The model under review builds one solid part; all positions refer to its coordinate system, in mm. A direction names the side the tool comes from. Round coordinates to 2 decimals unless told otherwise and drop trailing zeros. Write each loop counter-clockwise with the first axis right and the second up, starting at its lowest first coordinate (ties: lowest second). Pieces come first, ordered by that corner, then holes. Notation, with made-up numbers: (79, -21.75) -> (99, -21.75) arc R17 ccw to (99, 5.25) -> close; hole circle Ø10 at (81, -16). An arc over 180 degrees is marked (long way). Use CSV: the item, a comma, the result in double quotes. Start each with the question number.
1) Machinability: for faces 1 (the face through (29, 9, -4.8)), 2 (the face through (15, 2, -10)), 3 (the face through (-27.8, 2.74, 7.27)), which of the approach directions +Z, -Z, +X, -X, +Y, -Y give a long, thin tool a straight path to every point of the face, cutting with its end or side? Answer none if there is none.
2) Mouldability with a two-part tool opening along Z and no side actions: class faces 4 (the face through (-14.75, 0.56, -9.58)), 5 (the face through (-29.88, 14.56, -7.84)) as released by +Z, released by -Z, zero draft, split by the parting line, or undercut.
3) Take a section at C-C, the plane z = 17. Give the boundary of the cut face in (x, y).
4) For pin 1 Ø6 at (y, z) = (22, -5) entering from +X; pin 2 Ø5 at (x, z) = (-26, -3.5) entering from +Y; pin 3 Ø2.5 at (x, z) = (0, -8) entering from +Y; pin 4 Ø8 at (x, z) = (6, 9.5) entering from +Y, all flat-tipped, find the tip position at first contact; note any pin that passes through.
5) Wall thickness on probe 1 along Z at (x, y) = (0, 14); probe 2 along Z at (x, y) = (-22, 10); probe 3 along X at (y, z) = (9.5, -10.5): over which ranges is each line inside the solid? List them lowest first. Write a range as [from, to].
6) Take a section at D-D, the plane z = 12. Give the boundary of the cut face in (x, y).
7) Take a section at B-B, the plane y = 15. Give the boundary of the cut face in (x, z).
8) Take a section at A-A, the plane x = 0. Give the boundary of the cut face in (y, z).
from build123d import *

# Parameters (mm, degrees)
EXTRUDE_1_DEPTH     = 25
EXTRUDE_2_DEPTH     = 36
SKETCH_3_W          = 15
SKETCH_3_H          = 6
EXTRUDE_3_DEPTH     = 12
SKETCH_4_R          = 0.95
CUT_EXTRUDE_1_DEPTH = 21
SKETCH_5_R          = 4
SKETCH_5_R_2        = 1.45
EXTRUDE_4_DEPTH     = 23
SKETCH_6_R          = 1.75
CUT_EXTRUDE_2_DEPTH = 20
SKETCH_7_R          = 2.5
CUT_EXTRUDE_3_DEPTH = 2
CUT_EXTRUDE_4_DEPTH = 53.393911874
FILLET_4_R          = 1


with BuildPart() as part:
    # 草图1 → 凸台-拉伸1 (new, symmetric)
    with BuildSketch(Plane.XY):
        Polygon((0, 0), (9.650045346, 0), (39.194277936, -5.20944533), (39.888870647, -1.270214318), (10, 4), (0, 4), align=None)
    extrude_1 = extrude(amount=EXTRUDE_1_DEPTH, both=True)

    # 草图2 → 凸台-拉伸2 (add)
    with BuildSketch(Plane.XY.offset(25)):
        Polygon((20.192715587, 2.202749235), (20.513964715, 4.024643578), (35.286081011, 1.419920913), (34.964831882, -0.40197343), align=None)
    extrude_2 = extrude(amount=-EXTRUDE_2_DEPTH)

    # 草图3 → 凸台-拉伸3 (add)
    with BuildSketch(Plane(origin=(1.306826311, 7.411380301, 0), x_dir=(0.9848077530122079, -0.1736481776669312, 0), z_dir=(0.1736481776669312, 0.9848077530122079, 0))):
        with Locations((27.003439474, -22)):
            Rectangle(SKETCH_3_W, SKETCH_3_H)
        with Locations((27.003439474, 7.8)):
            Rectangle(SKETCH_3_W, SKETCH_3_H)
    extrude_3 = extrude(amount=EXTRUDE_3_DEPTH)

    # 草图4 → 切除-拉伸1 (cut)
    with BuildSketch(Plane(origin=(33.979254699, -5.991459388, 0), x_dir=(0, 0, -1), z_dir=(0.9848077530122081, -0.17364817766693072, 0))):
        with Locations(Location((-20.95, 14.025712789, 0), (0, 0, 90))):
            Circle(SKETCH_4_R)
        with Locations(Location((6.75, 14.025712789, 0), (0, 0, 90))):
            Circle(SKETCH_4_R)
    cut_extrude_1 = extrude(amount=-CUT_EXTRUDE_1_DEPTH, mode=Mode.SUBTRACT)

    # 镜向1: 凸台-拉伸1, 凸台-拉伸2, 凸台-拉伸3, 切除-拉伸1 across plane
    add(extrude_1.mirror(Plane(origin=(0, 0, 0), x_dir=(0, 0, 1), z_dir=(1, 0, 0))))
    add(extrude_2.mirror(Plane(origin=(0, 0, 0), x_dir=(0, 0, 1), z_dir=(1, 0, 0))))
    add(extrude_3.mirror(Plane(origin=(0, 0, 0), x_dir=(0, 0, 1), z_dir=(1, 0, 0))))
    add(cut_extrude_1.mirror(Plane(origin=(0, 0, 0), x_dir=(0, 0, 1), z_dir=(1, 0, 0))), mode=Mode.SUBTRACT)

    # 草图5 → 凸台-拉伸4 (add)
    # profile 1 of 2: a face of its own
    with BuildSketch(Plane(origin=(0, 4, 0), x_dir=(1, 0, 0), z_dir=(0, 1, 0))):
        with Locations((0, -12)):
            Circle(SKETCH_5_R)
        with Locations(Location((0, -12, 0), (0, 0, 180))):
            Circle(SKETCH_5_R_2, mode=Mode.SUBTRACT)
    # profile 2 of 2: a face of its own
    with BuildSketch(Plane(origin=(0, 4, 0), x_dir=(1, 0, 0), z_dir=(0, 1, 0))):
        with Locations((0, 8)):
            Circle(SKETCH_5_R)
        with Locations(Location((0, 8, 0), (0, 0, 180))):
            Circle(SKETCH_5_R_2, mode=Mode.SUBTRACT)
    extrude(amount=EXTRUDE_4_DEPTH)

    # 草图6 → 切除-拉伸2 (cut)
    with BuildSketch(Plane(origin=(0, 4, 0), x_dir=(1, 0, 0), z_dir=(0, 1, 0))):
        with Locations(Location((0, -20, 0), (0, 0, 180))):
            Circle(SKETCH_6_R)
        with Locations((-13, 9.5)):
            Circle(SKETCH_6_R)
        with Locations(Location((13, 9.5, 0), (0, 0, 180))):
            Circle(SKETCH_6_R)
    extrude(amount=-CUT_EXTRUDE_2_DEPTH, mode=Mode.SUBTRACT)

    # 草图7 → 切除-拉伸3 (cut)
    with BuildSketch(Plane(origin=(0, 4, 0), x_dir=(1, 0, 0), z_dir=(0, 1, 0))):
        with Locations(Location((-13, 9.5, 0), (0, 0, 180))):
            Circle(SKETCH_7_R)
        with Locations(Location((13, 9.5, 0), (0, 0, 180))):
            Circle(SKETCH_7_R)
    extrude(amount=-CUT_EXTRUDE_3_DEPTH, mode=Mode.SUBTRACT)

    # 草图8 → 切除-拉伸4 (cut, through all)
    with BuildSketch(Plane(origin=(0, 4, 0), x_dir=(1, 0, 0), z_dir=(0, 1, 0))):
        Polygon((-4, 23), (-1, 23), (-1, 25), (1, 25), (1, 23), (4, 23), (4, 14), (-4, 14), align=None)
    extrude(amount=-CUT_EXTRUDE_4_DEPTH, mode=Mode.SUBTRACT)

    # 圆角4
    fillet_4_edges = [part.edges().sort_by_distance(p)[0] for p in [
        (4, 2, -23),
        (4, 2, -14),
        (-4, 2, -14),
        (-4, 2, -23),
        (1, 2, -23),
        (-1, 2, -23),
    ]]
    fillet(fillet_4_edges, radius=FILLET_4_R)


solid = part.part
Values found:
1,face 1,"+X, +Y"
1,face 2,"+Y"
1,face 3,"-X, +Y"
2,face 4,"undercut"
2,face 5,"zero draft"
3,outline,"(-39.89, -1.27) -> (-39.19, -5.21) -> (-9.65, 0) -> (9.65, 0) -> (39.19, -5.21) -> (39.89, -1.27) -> (34.96, -0.4) -> (35.29, 1.42) -> (20.51, 4.02) -> (20.19, 2.2) -> (10, 4) -> (-10, 4) -> (-20.19, 2.2) -> (-20.51, 4.02) -> (-35.29, 1.42) -> (-34.96, -0.4) -> close"
4,pin 1,"x = 4"
4,pin 2,"y = 15.62"
4,pin 3,"y = 4"
4,pin 4,"y = 27"
5,probe 1,"[-12, -9.45], [-6.55, -4], [8, 10.55], [13.45, 16]"
5,probe 2,"[-10.8, -7.63], [-5.87, -4.8], [19, 20.07], [21.83, 25]"
5,probe 3,"[-36.71, -21.48], [-3.12, 3.12], [21.48, 36.71]"
6,outline,"(-39.89, -1.27) -> (-39.19, -5.21) -> (-9.65, 0) -> (9.65, 0) -> (39.19, -5.21) -> (39.89, -1.27) -> (34.96, -0.4) -> (35.29, 1.42) -> (20.51, 4.02) -> (20.19, 2.2) -> (10, 4) -> (4, 4) -> (4, 27) -> (1.45, 27) -> (1.45, 4) -> (-1.45, 4) -> (-1.45, 27) -> (-4, 27) -> (-4, 4) -> (-10, 4) -> (-20.19, 2.2) -> (-20.51, 4.02) -> (-35.29, 1.42) -> (-34.96, -0.4) -> close"
7,outline,"(-27.37, -10.8) -> (-22.45, -10.8) -> (-22.45, -4.8) -> (-27.37, -4.8) -> close; (-27.37, 19) -> (-22.45, 19) -> (-22.45, 25) -> (-27.37, 25) -> close; circle Ø8 at (0, -8); circle Ø8 at (0, 12); (22.45, -10.8) -> (27.37, -10.8) -> (27.37, -4.8) -> (22.45, -4.8) -> close; (22.45, 19) -> (27.37, 19) -> (27.37, 25) -> (22.45, 25) -> close; hole circle Ø2.9 at (0, -8); hole circle Ø2.9 at (0, 12)"
8,outline,"(0, -14) -> (4, -14) -> (4, -12) -> (27, -12) -> (27, -9.45) -> (4, -9.45) -> (4, -6.55) -> (27, -6.55) -> (27, -4) -> (4, -4) -> (4, 8) -> (27, 8) -> (27, 10.55) -> (4, 10.55) -> (4, 13.45) -> (27, 13.45) -> (27, 16) -> (4, 16) -> (4, 18.25) -> (0, 18.25) -> close; (0, 21.75) -> (4, 21.75) -> (4, 25) -> (0, 25) -> close"
